Part model, mm, in its own coordinate system. Face numbers are marked on the shaded views. A direction names the side the tool comes from. Give positions to 0.01 mm unless a question says otherwise; leave off trailing zeros. Write each loop counter-clockwise with the first axis right and the second up, starting at its lowest first coordinate (ties: lowest second). Pieces come first, ordered by that corner, then holes. Notation, with made-up numbers: M -38.75,47 L -2.75,47 A8 ccw -2.75,60 Z; hole C 77,45 d1. An arc over 180 degrees is marked long. Use CSV: the item, a comma, the result in double quotes. Start each with the question number.
1. Mould opens along X. For the marked faces 3, 4, 5 and 6 say: pulls with the +X half, pulls with the -X half, needs draft (parallel to the pull), parting line crosses it, or undercut.
2. Band-saw the part on C-C, the plane z = 18. List the corners of the cut face in (x, y).
3. Drop flat-ended pins along their axis: pin 1 Ø4.5 at (y, z) = (0, 170) entering from +X; pin 2 Ø1 at (y, z) = (-122, 133) entering from -X; pin 3 Ø12 at (x, z) = (-13, 157) entering from -Y; pin 4 Ø12 at (x, z) = (10, 238.5) entering from +Y. Give the stop position or say it passes through.
4. Drill centre lines: line 1 along Z through (x, y) = (18, 0); line 2 along X through (y, z) = (-11, 66); line 3 along X through (y, z) = (0, 105). Where is each one in solid material? Low to high. Write a range as from..to.
5. 3-axis set-ups, long thin cutter, end or side, ignore diameter. For the marked faces 1 and 2: which of +Z, -Z, +X, -X, +Y, -Y reach the whole face in a straight line?
6. Band-saw the part on D-D, the plane y = -200. List the corners of the cut face in (x, z), then the cut area to 3 significant figures.
7. Band-saw the part on B-B, the plane y = -50. List the corners of the cut face in (x, z).
8. Band-saw the part on A-A, the plane z = 70. List the corners of the cut face in (x, y).
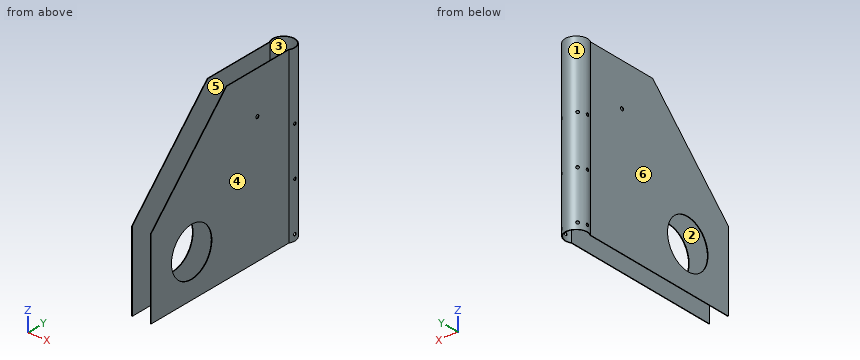
from build123d import *

# Parameters (mm, degrees)
F3_DEPTH  = 280
F4_DEPTH  = 280
F5_R      = 2.4
F6_DEPTH  = 18.5
F8_DEPTH  = 25
F10_R     = 2.4
F11_DEPTH = 25
F12_R     = 40
F12_R_2   = 3
F13_DEPTH = 20


with BuildPart() as f3:
    # F2 (on Top) → F3 (new body)
    with BuildSketch(Plane.XY):
        with BuildLine():
            ThreePointArc((16, -9.2870878105), (0, 18.5), (-16, -9.2870878105))
            Line((-16, -9.2870878105), (-16, -18.5))
            Line((-16, -18.5), (-16, -281.5))
            Line((-16, -281.5), (16, -281.5))
            Line((16, -281.5), (16, -18.5))
            Line((16, -18.5), (16, -9.2870878105))
        make_face()
    extrude(amount=F3_DEPTH)

    # F0 (on Top) → F4 (cut)
    with BuildSketch(Plane.XY):
        with BuildLine():
            Line((15, -17.5), (15, -9.0138781887))
            ThreePointArc((15, -9.0138781887), (0, 17.5), (-15, -9.0138781887))
            Line((-15, -9.0138781887), (-15, -17.5))
            Line((-15, -17.5), (-15, -282.5))
            Line((-15, -282.5), (15, -282.5))
            Line((15, -282.5), (15, -17.5))
        make_face()
    extrude(amount=F4_DEPTH, mode=Mode.SUBTRACT)

    # F5 (on Right) → F6 (cut, symmetric)
    with BuildSketch(Plane.YZ):
        with Locations((0, 170)):
            Circle(F5_R)
        with Locations((0, 90)):
            Circle(F5_R)
        with Locations((0, 10)):
            Circle(F5_R)
    extrude(amount=F6_DEPTH, both=True, mode=Mode.SUBTRACT)

    # F7 (on face) → F8 (cut)
    with BuildSketch(Plane(origin=(0, 0, 0), x_dir=(0.7071067812, -0.7071067812, 0), z_dir=(-0.7071067812, -0.7071067812, 0))):
        with BuildLine():
            ThreePointArc((2.4, 10), (0, 12.4), (-2.4, 10))
            Line((-2.4, 10), (2.4, 10))
        make_face()
        with BuildLine():
            Line((2.4, 10), (-2.4, 10))
            ThreePointArc((-2.4, 10), (0, 7.6), (2.4, 10))
        make_face()
        with BuildLine():
            ThreePointArc((-2.4, 90), (0, 87.6), (2.4, 90))
            Line((2.4, 90), (-2.4, 90))
        make_face()
        with BuildLine():
            Line((-2.4, 90), (2.4, 90))
            ThreePointArc((2.4, 90), (0, 92.4), (-2.4, 90))
        make_face()
        with BuildLine():
            ThreePointArc((-2.4, 170), (0, 167.6), (2.4, 170))
            Line((2.4, 170), (-2.4, 170))
        make_face()
        with BuildLine():
            Line((-2.4, 170), (2.4, 170))
            ThreePointArc((2.4, 170), (0, 172.4), (-2.4, 170))
        make_face()
    extrude(amount=-F8_DEPTH, mode=Mode.SUBTRACT)

    # F10 (on face) → F11 (cut)
    with BuildSketch(Plane(origin=(0, 0, 0), x_dir=(0.7071067812, 0.7071067812, 0), z_dir=(0.7071067812, -0.7071067812, 0))):
        with Locations((0, 170)):
            Circle(F10_R)
        with Locations((0, 90)):
            Circle(F10_R)
        with Locations((0, 10)):
            Circle(F10_R)
    extrude(amount=-F11_DEPTH, mode=Mode.SUBTRACT)

    # F12 (on Right) → F13 (cut, symmetric)
    with BuildSketch(Plane.YZ):
        with Locations((-201.2879049778, 70)):
            Circle(F12_R)
        Polygon((-131.954, 280), (-281.954, 280), (-281.954, 130), align=None)
        with Locations((-71.2879049778, 210)):
            Circle(F12_R_2)
    extrude(amount=F13_DEPTH, both=True, mode=Mode.SUBTRACT)


solid = f3.part
Output:
1,face 3,"undercut"
1,face 4,"pulls with the +X half"
1,face 5,"undercut"
1,face 6,"pulls with the -X half"
2,outline,"M -16,-281.5 L -15,-281.5 L -15,-9.01 A17.5 cw long 15,-9.01 L 15,-281.5 L 16,-281.5 L 16,-9.29 A18.5 ccw long -16,-9.29 Z"
3,pin 1,"passes through"
3,pin 2,"stops at x = -16"
3,pin 3,"stops at y = -260.61"
3,pin 4,"stops at y = 18.06"
4,line 1,"z = 0..7.6, 12.4..87.6, 92.4..167.6, 172.4..280"
4,line 2,"x = -16..-15, 15..16"
4,line 3,"x = -18.5..-17.5, 17.5..18.5"
5,face 1,"+Z, -Z"
5,face 2,"+Z, -Z, -Y"
6,outline,"M -16,0 L -15,0 L -15,30.02 L -16,30.02 Z; M -16,109.98 L -15,109.98 L -15,211.95 L -16,211.95 Z; M 15,0 L 16,0 L 16,30.02 L 15,30.02 Z; M 15,109.98 L 16,109.98 L 16,211.95 L 15,211.95 Z"
6,area,"264 mm²"
7,outline,"M -16,0 L -15,0 L -15,280 L -16,280 Z; M 15,0 L 16,0 L 16,280 L 15,280 Z"
8,outline,"M -16,-281.5 L -15,-281.5 L -15,-241.29 L -16,-241.29 Z; M -16,-161.29 L -15,-161.29 L -15,-9.01 A17.5 cw long 15,-9.01 L 15,-161.29 L 16,-161.29 L 16,-9.29 A18.5 ccw long -16,-9.29 Z; M 15,-281.5 L 16,-281.5 L 16,-241.29 L 15,-241.29 Z"
